The model under review builds one solid part; all positions refer to its coordinate system, in mm. Face numbers are marked on the shaded views. Coordinates: 2 decimals unless noted, no trailing zeros. Order: outer loops, then holes, each group sorted by start corner. A loop starts at its lowest first (then second) coordinate and runs counter-clockwise, first axis right, second up.
from build123d import *

# Parameters (mm, degrees)
SKETCH1_R           = 45.85
SKETCH1_R_2         = 1.5635
SKETCH1_R_3         = 39.3
BOSS_EXTRUDE1_DEPTH = 6
BOSS_EXTRUDE2_START = 3
SKETCH1_4_R         = 45.85
SKETCH1_4_R_2       = 27.9
SKETCH1_4_R_3       = 1.5635
BOSS_EXTRUDE2_DEPTH = 3
SKETCH2_R           = 3
CUT_EXTRUDE1_DEPTH  = 3


with BuildPart() as part:
    # Sketch1 → Boss-Extrude1 (new body)
    with BuildSketch(Plane(origin=(0, 0, 0), x_dir=(1, 0, 0), z_dir=(0, 1, 0))):
        with Locations(Location((0, 0, 0), (0, 0, 270))):
            Circle(SKETCH1_R)
        with Locations(Location((42.5, 0, 0), (0, 0, 270))):
            Circle(SKETCH1_R_2, mode=Mode.SUBTRACT)
        with Locations(Location((-21.25, -36.806079661, 0), (0, 0, 270))):
            Circle(SKETCH1_R_2, mode=Mode.SUBTRACT)
        with Locations(Location((-21.25, 36.806079661, 0), (0, 0, 270))):
            Circle(SKETCH1_R_2, mode=Mode.SUBTRACT)
        with Locations(Location((0, 0, 0), (0, 0, 270))):
            Circle(SKETCH1_R_3, mode=Mode.SUBTRACT)
    extrude(amount=-BOSS_EXTRUDE1_DEPTH)

    # Sketch1_4 → Boss-Extrude2 (add)
    with BuildSketch(Plane(origin=(0, 0, 0), x_dir=(1, 0, 0), z_dir=(0, 1, 0)).offset(BOSS_EXTRUDE2_START)):
        with Locations(Location((0, 0, 0), (0, 0, 270))):
            Circle(SKETCH1_4_R)
        with Locations(Location((0, 0, 0), (0, 0, 270))):
            Circle(SKETCH1_4_R_2, mode=Mode.SUBTRACT)
        with Locations(Location((42.5, 0, 0), (0, 0, 270))):
            Circle(SKETCH1_4_R_3, mode=Mode.SUBTRACT)
        with Locations(Location((-21.25, -36.806079661, 0), (0, 0, 270))):
            Circle(SKETCH1_4_R_3, mode=Mode.SUBTRACT)
        with Locations(Location((-21.25, 36.806079661, 0), (0, 0, 270))):
            Circle(SKETCH1_4_R_3, mode=Mode.SUBTRACT)
    extrude(amount=-BOSS_EXTRUDE2_DEPTH)

    # Sketch2 → Cut-Extrude1 (cut)
    with BuildSketch(Plane(origin=(0, 3, 0), x_dir=(1, 0, 0), z_dir=(0, 1, 0))):
        with Locations(Location((42.5, 0, 0), (0, 0, 270))):
            Circle(SKETCH2_R)
        with Locations(Location((-21.25, -36.806079661, 0), (0, 0, 270))):
            Circle(SKETCH2_R)
        with Locations(Location((-21.25, 36.806079661, 0), (0, 0, 270))):
            Circle(SKETCH2_R)
    extrude(amount=-CUT_EXTRUDE1_DEPTH, mode=Mode.SUBTRACT)


solid = part.part
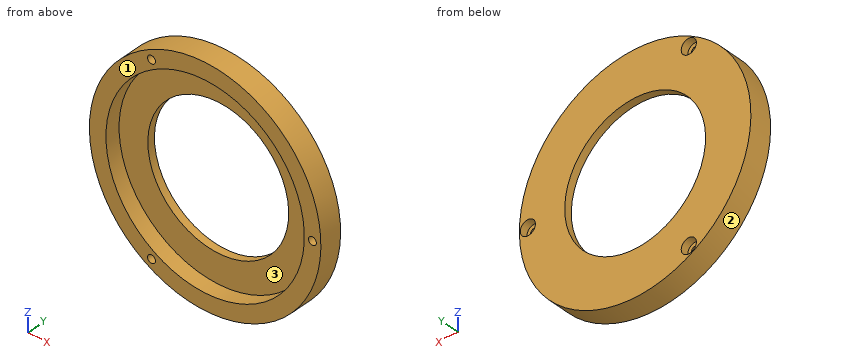
(1) Consider section C-C (z = 0). Give the boundary of the cut face in (x, y), then the cut area to 3 significant figures.
(2) Consider section D-D (z = 10). Give the boundary of the cut face in (x, y), then the cut area to 3 significant figures.
(3) Wall thickness on line 1 (X direction, y = 1.5, z = 0); line 2 (Y direction, x = 9, z = 38); line 3 (Z direction, x = 20.5, y = 0.5): over which ranges is each line inside the solid? List them lowest first.
(4) Consider section B-B (y = 1.75). Give the boundary of the cut face in (x, z), then the cut area to 3 significant figures.
(5) Insertion check: pin 1 Ø6.5 at (x, z) = (-22.5, 36.5) entering from +Y; pin 2 Ø5 at (x, z) = (-21.25, 36.81) entering from +Y; pin 3 Ø1 at (y, z) = (0.5, 16.5) entering from -X; pin 4 Ø5 at (x, z) = (-27, -9) entering from -Y. Each pin has a flat end and moves straight along its axis. Give the tip position at first contact, or say it passes through.
(6) The part is to be moulded in two halves that separate along Z. For the marked faces 1, 2 and 3, say which applies: +Z half, -Z half, draft (parallel to the pull), parting line (faces both ways), or undercut.
(7) Consider section A-A (x = 0). Give the boundary of the cut face in (y, z).
Findings:
1. outline: (-45.85, -6) - (-39.3, -6) - (-39.3, 0) - (-27.9, 0) - (-27.9, 3) - (-45.85, 3) - close; (27.9, 0) - (39.3, 0) - (39.3, -6) - (40.94, -6) - (40.94, 0) - (39.5, 0) - (39.5, 3) - (27.9, 3) - close; (44.06, -6) - (45.85, -6) - (45.85, 3) - (45.5, 3) - (45.5, 0) - (44.06, 0) - close
1. area: 150 mm2
2. outline: (-44.75, -6) - (-38.01, -6) - (-38.01, 0) - (-26.05, 0) - (-26.05, 3) - (-44.75, 3) - close; (26.05, 0) - (38.01, 0) - (38.01, -6) - (44.75, -6) - (44.75, 3) - (26.05, 3) - close
2. area: 193 mm2
3. line 1: x = -45.85 to -27.9, 27.9 to 39.5, 45.5 to 45.85
3. line 2: y = 0 to 3
3. line 3: z = -41.01 to -18.93, 18.93 to 41.01
4. outline: circle Ø91.7 at (0, 0); hole circle Ø55.8 at (0, 0); hole circle Ø6 at (-21.25, -36.81); hole circle Ø6 at (-21.25, 36.81); hole circle Ø6 at (42.5, 0)
4. area: 4,070 mm2
5. pin 1: stops at y = 3
5. pin 2: stops at y = 0
5. pin 3: stops at x = -42.97
5. pin 4: stops at y = 0
6. face 1: draft
6. face 2: parting line
6. face 3: undercut
7. outline: (-6, -45.85) - (3, -45.85) - (3, -27.9) - (0, -27.9) - (0, -39.3) - (-6, -39.3) - close; (-6, 39.3) - (0, 39.3) - (0, 27.9) - (3, 27.9) - (3, 45.85) - (-6, 45.85) - close
